from build123d import *

# Parameters (mm, degrees)
SKETCH_1_R          = 2
EXTRUDE_1_DEPTH     = 8
SKETCH_2_R          = 3.75
EXTRUDE_2_DEPTH     = 5
CUT_EXTRUDE_2_DEPTH = 3
FILLET_1_R          = 0.5


with BuildPart() as part:
    # 草图1 → 凸台-拉伸1 (new body)
    with BuildSketch(Plane.XY):
        Circle(SKETCH_1_R)
    extrude(amount=EXTRUDE_1_DEPTH)

    # 草图2 → 凸台-拉伸2 (add)
    with BuildSketch(Plane(origin=(0, 0, 0), x_dir=(-1, 0, 0), z_dir=(0, 0, -1))):
        Circle(SKETCH_2_R)
    extrude(amount=EXTRUDE_2_DEPTH)

    # 草图4 → 切除-拉伸2 (cut)
    with BuildSketch(Plane(origin=(0, 0, -5), x_dir=(-1, 0, 0), z_dir=(0, 0, -1))):
        Polygon((-1.4, 2.424871131), (1.4, 2.424871131), (2.8, 0), (1.4, -2.424871131), (-1.4, -2.424871131), (-2.8, 0), align=None)
    extrude(amount=-CUT_EXTRUDE_2_DEPTH, mode=Mode.SUBTRACT)

    # 圆角1
    fillet_1_edges = [part.edges().sort_by_distance(p)[0] for p in [
        (-1.4, 2.424871131, -3.5),
        (-2.8, 0, -3.5),
        (-1.4, -2.424871131, -3.5),
        (1.4, -2.424871131, -3.5),
        (2.8, 0, -3.5),
        (1.4, 2.424871131, -3.5),
        (-2, 0, 8),
        (3.75, 0, 0),
        (3.75, 0, -5),
    ]]
    fillet(fillet_1_edges, radius=FILLET_1_R)


solid = part.part
Source: CAD feature listing. Evaluate the final solid. Frame: model axes, mm. A direction names the side the tool comes from. Round coordinates to 2 decimals unless told otherwise and drop trailing zeros. Loops run counter-clockwise (first coordinate to the right, second up) from the corner with the lowest first, then second, coordinate; pieces in that order, holes last. Notation, with made-up numbers: (61, 83) -> (68, 83) arc R19 ccw to (68, 98) -> close; hole circle Ø11 at (-11.75, 1). An arc over 180 degrees is marked (long way). Answer as a JSON object with one key per item and string values. Group by question number.
Q1. Section query A-A (x = 0). Output: boundary loops of the cut face in (y, z), plus the area to 3 significant figures.
Q2. Access query for faces 1 (the flat face through (0, 0, -2)), 2 (the cylindrical face through (0, -2, 4)), 3 (the flat face through (0, 0, 8)). Directions: +Z, -Z, +X, -X, +Y, -Y. A direction counts if a zero-diameter tool reaches every point of the face in a straight line with its end or side. Return the directions, or none.
Q3. Mould query, pull axis X, two halves, no side actions, for faces 4 (the flat face through (-2.09, 1.23, -3.52)), 5 (the flat face through (2, -2, -5)), 6 (the cylindrical face through (3.746, 0.165, -2.472)). Classes: pulls with the +X half, pulls with the -X half, needs draft (parallel to the pull), parting line crosses it, or undercut.
Q4. Contact query for flat-ended pins moving along their axis: P1, Ø1.5, axis at y = -3, z = 2.5, coming from the +X side; P2, Ø2.5, axis at x = -0.5, z = -4, coming from the +Y side; P3, Ø2, axis at x = -3, z = -3.5, coming from the +Y side; P4, Ø1.5, axis at y = -1, z = -0.5, coming from the -X side. Output: stop coordinate, or through.
Q5. Ray query, line 1 (Z direction, x = -3, y = -0.5); line 2 (Z direction, x = 1.5, y = -1.5); line 3 (X direction, y = 0.25, z = -4). Return the intervals inside material, ascending. Write a range as from..to.
Q6. Section query D-D (z = -0.75). Output: boundary loops of the cut face in (x, y).
Q7. Section query C-C (y = 0). Output: boundary loops of the cut face in (x, z), plus the area to 3 significant figures.
Q8. Section query B-B (z = -3.75). Output: boundary loops of the cut face in (x, y), plus the area to 3 significant figures.
Completed:
{
 "1": {"outline": "(-3.75, -4.5) arc R0.5 ccw to (-3.25, -5) -> (-2.42, -5) -> (-2.42, -2) -> (2.42, -2) -> (2.42, -5) -> (3.25, -5) arc R0.5 ccw to (3.75, -4.5) -> (3.75, -0.5) arc R0.5 ccw to (3.25, 0) -> (2, 0) -> (2, 7.5) arc R0.5 ccw to (1.5, 8) -> (-1.5, 8) arc R0.5 ccw to (-2, 7.5) -> (-2, 0) -> (-3.25, 0) arc R0.5 ccw to (-3.75, -0.5) -> close", "area": "54.6 mm²"},
 "2": {"face 1": "-Z", "face 2": "+Z", "face 3": "+Z, +X, -X, +Y, -Y"},
 "3": {"face 4": "undercut", "face 5": "needs draft", "face 6": "parting line crosses it"},
 "4": {"P1": "through", "P2": "y = 3.75", "P3": "y = 3.17", "P4": "x = -3.74"},
 "5": {"line 1": "-5..0", "line 2": "-2..0", "line 3": "-3.74..-2.66, 2.66..3.74"},
 "6": {"outline": "circle Ø7.5 at (0, 0)"},
 "7": {"outline": "(-3.75, -4.5) arc R0.5 ccw to (-3.25, -5) -> (-2.72, -5) -> (-2.72, -2) -> (2.72, -2) -> (2.72, -5) -> (3.25, -5) arc R0.5 ccw to (3.75, -4.5) -> (3.75, -0.5) arc R0.5 ccw to (3.25, 0) -> (2, 0) -> (2, 7.5) arc R0.5 ccw to (1.5, 8) -> (-1.5, 8) arc R0.5 ccw to (-2, 7.5) -> (-2, 0) -> (-3.25, 0) arc R0.5 ccw to (-3.75, -0.5) -> close", "area": "52.8 mm²"},
 "8": {"outline": "circle Ø7.5 at (0, 0); hole (-2.66, -0.25) -> (-1.54, -2.17) arc R0.5 ccw to (-1.11, -2.42) -> (1.11, -2.42) arc R0.5 ccw to (1.54, -2.17) -> (2.66, -0.25) arc R0.5 ccw to (2.66, 0.25) -> (1.54, 2.17) arc R0.5 ccw to (1.11, 2.42) -> (-1.11, 2.42) arc R0.5 ccw to (-1.54, 2.17) -> (-2.66, 0.25) arc R0.5 ccw to start", "area": "23.9 mm²"}
}
